Design review of the part shown in the three views and the two pictorial views. Dimensions are in mm from the part's minimum x, y and z. A direction names the side the tool comes from. Coordinates: 2 decimals unless noted, no trailing zeros. Write each loop counter-clockwise with the first axis right and the second up, starting at its lowest first coordinate (ties: lowest second). Pieces come first, ordered by that corner, then holes. Notation, with made-up numbers: (-34, 41.5) - (19, 41.5) arc R14 ccw to (19, 45.5) - close; hole circle Ø2 at (44, 79.25). An arc over 180 degrees is marked (long way). Answer as CSV lines item,"result". Start each with the question number.
Q1. Machinability: for the marked faces 5, 6, 7 and 8, which of the approach directions +Z, -Z, +X, -X, +Y, -Y give a long, thin tool a straight path to every point of the face, cutting with its end or side? Answer none if there is none.
Q2. We need section A-A (x = 27.5). Write out the cut boundary in (y, z), plus the area to 3 significant figures.
Q3. Clearance check with flat-ended pins moving along their axes: pin 1 (12 mm diameter, centred on y = 18, z = 16, fed in from +X); pin 2 (3 mm diameter, centred on x = 24.5, y = 61.5, fed in from -Z); pin 3 (7.5 mm diameter, centred on y = 4.5, z = 34, fed in from -X); pin 4 (3 mm diameter, centred on x = 6, z = 3, fed in from +Y). State where each tip first meets the part, or that it passes through.
Q4. Mouldability with a two-part tool opening along Z and no side actions: class the marked faces 1, 2, 3 and 4 as pulls with the +Z half, pulls with the -Z half, needs draft (parallel to the pull), parting line crosses it, or undercut.
Q5. We need section D-D (x = 14.5). Write out the cut boundary in (y, z).
Q6. For line 1 along X through (y, z) = (61.5, 29); line 2 along Y through (x, z) = (24.5, 23.5); line 3 along Y through (x, z) = (14.5, 27.75), list the stretches that pass through material, from the lowest coordinate up. Write a range as [from, to].
Q7. We need section C-C (z = 26). Write out the cut boundary in (x, y).
Q8. We need section B-B (z = 36.5). Write out the cut boundary in (x, y), plus the area to 3 significant figures.
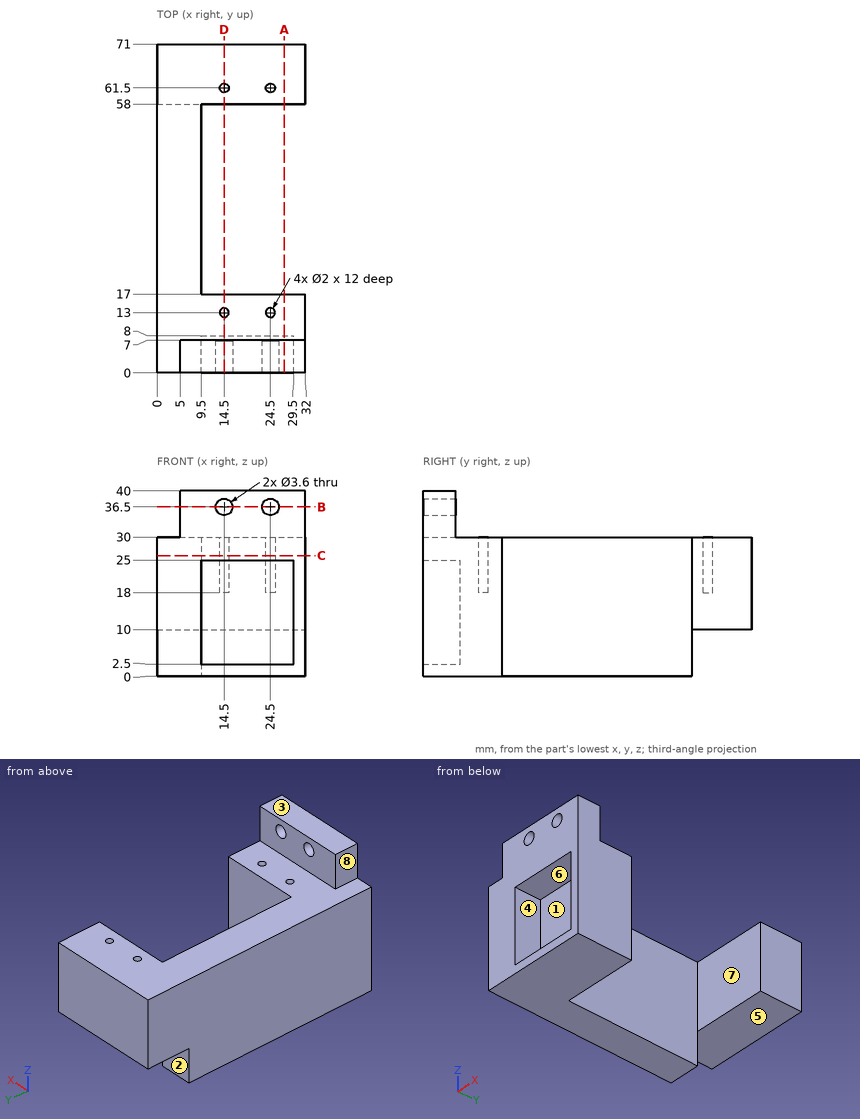
Results list:
1,face 5,"-Z, +X, -X, +Y"
1,face 6,"-Y"
1,face 7,"+Z, -Z, +X"
1,face 8,"+Z, -X, +Y, -Y"
2,outline,"(0, 0) - (17, 0) - (17, 30) - (7, 30) - (7, 40) - (0, 40) - (0, 25) - (8, 25) - (8, 2.5) - (0, 2.5) - close; (58, 10) - (71, 10) - (71, 30) - (58, 30) - close"
2,area,"660 mm2"
3,pin 1,"stops at x = 32"
3,pin 2,"stops at z = 10"
3,pin 3,"stops at x = 5"
3,pin 4,"stops at y = 58"
4,face 1,"undercut"
4,face 2,"needs draft"
4,face 3,"pulls with the +Z half"
4,face 4,"undercut"
5,outline,"(0, 0) - (17, 0) - (17, 30) - (14, 30) - (14, 18) - (12, 18) - (12, 30) - (7, 30) - (7, 34.7) - (0, 34.7) - (0, 25) - (8, 25) - (8, 2.5) - (0, 2.5) - close; (0, 38.3) - (7, 38.3) - (7, 40) - (0, 40) - close; (58, 10) - (71, 10) - (71, 30) - (62.5, 30) - (62.5, 18) - (60.5, 18) - (60.5, 30) - (58, 30) - close"
6,line 1,"x = [0, 13.5], [15.5, 23.5], [25.5, 32]"
6,line 2,"y = [8, 12], [14, 17], [58, 60.5], [62.5, 71]"
6,line 3,"y = [0, 12], [14, 17], [58, 60.5], [62.5, 71]"
7,outline,"(0, 0) - (32, 0) - (32, 17) - (9.5, 17) - (9.5, 58) - (32, 58) - (32, 71) - (0, 71) - close; hole circle Ø2 at (14.5, 13); hole circle Ø2 at (14.5, 61.5); hole circle Ø2 at (24.5, 13); hole circle Ø2 at (24.5, 61.5)"
8,outline,"(5, 0) - (12.7, 0) - (12.7, 7) - (5, 7) - close; (16.3, 0) - (22.7, 0) - (22.7, 7) - (16.3, 7) - close; (26.3, 0) - (32, 0) - (32, 7) - (26.3, 7) - close"
8,area,"139 mm2"
